```python
from build123d import *

# Parameters (mm, degrees)
F0_W     = 444.5
F0_H     = 654.05
F1_DEPTH = 1092.2
F2_W     = 381
F2_H     = 304.8
F3_DEPTH = 654.05
F5_DEPTH = 304.801
F7_DEPTH = 482.6


# Not quite as in the source:
# - a pattern or mirror of a feature is missing from the dataset's text; its kind, count and spacing are read off the source's solid


with BuildPart() as f1:
    # F0 (on Top) → F1 (new body)
    with BuildSketch(Plane.XY):
        Rectangle(F0_W, F0_H)
    extrude(amount=F1_DEPTH)

    # F2 (on face) → F3 (join, through all)
    with BuildSketch(Plane.XZ.offset(327.025)):
        with Locations((412.75, 152.4)):
            Rectangle(F2_W, F2_H)
        with Locations((-412.75, 152.4)):
            Rectangle(F2_W, F2_H)
    extrude(amount=-F3_DEPTH)

    # F4 (on face) → F5 (cut, through all)
    with BuildSketch(Plane.XY.offset(304.8)):
        Polygon((-314.325, -234.95), (-314.325, 168.9629166667), (-511.175, -168.9629166667), (-511.175, -234.95), align=None)
        Polygon((-511.175, -168.9629166667), (-314.325, 168.9629166667), (-314.325, 234.95), (-511.175, 234.95), align=None)
    f5 = extrude(amount=-F5_DEPTH, mode=Mode.SUBTRACT)

    # F5_copies: F5 across plane
    add(f5.mirror(Plane(origin=(0, 0, 0), x_dir=(0, 0, 1), z_dir=(1, 0, 0))), mode=Mode.SUBTRACT)

    # F6 (on face) → F7 (cut)
    with BuildSketch(Plane.XZ.offset(327.025)):
        with BuildLine():
            ThreePointArc((82.55, 920.75), (58.3716647869, 979.121664787), (0, 1003.3))
            Line((0, 1003.3), (0, 920.75))
            Line((0, 920.75), (82.55, 920.75))
        make_face()
        with BuildLine():
            Line((0, 920.75), (0, 1003.3))
            ThreePointArc((0, 1003.3), (-58.371664787, 979.1216647869), (-82.55, 920.75))
            Line((-82.55, 920.75), (0, 920.75))
        make_face()
        with BuildLine():
            Line((82.55, 920.75), (0, 920.75))
            Line((0, 920.75), (0, 838.2))
            ThreePointArc((0, 838.2), (58.3716647869, 862.378335213), (82.55, 920.75))
        make_face()
        with BuildLine():
            Line((0, 838.2), (0, 920.75))
            Line((0, 920.75), (-82.55, 920.75))
            ThreePointArc((-82.55, 920.75), (-58.371664787, 862.3783352131), (0, 838.2))
        make_face()
        with BuildLine():
            Line((82.55, 787.4), (82.55, 920.75))
            ThreePointArc((82.55, 920.75), (58.3716647869, 862.378335213), (0, 838.2))
            Line((0, 838.2), (0, 787.4))
            Line((0, 787.4), (82.55, 787.4))
        make_face()
        with BuildLine():
            ThreePointArc((0, 838.2), (-58.371664787, 862.3783352131), (-82.55, 920.75))
            Line((-82.55, 920.75), (-82.55, 787.4))
            Line((-82.55, 787.4), (0, 787.4))
            Line((0, 787.4), (0, 838.2))
        make_face()
    extrude(amount=-F7_DEPTH, mode=Mode.SUBTRACT)


solid = f1.part
```
Geometry: final body of the model. Coordinates: model frame, mm. A direction names the side the tool comes from. Round coordinates to 2 decimals unless told otherwise and drop trailing zeros. Order: outer loops, then holes, each group sorted by start corner. A loop starts at its lowest first (then second) coordinate and runs counter-clockwise, first axis right, second up. Notation, with made-up numbers: (79, 11) -> (138, 11) arc R15 ccw to (138, 26) -> close; hole circle Ø3 at (52.25, 68.25). An arc over 180 degrees is marked (long way). Use CSV: the item, a comma, the result in double quotes. Start each with the question number.
1) First-contact query: pin 1 Ø12 at (y, z) = (-214.5, 953.5) entering from -X; pin 2 Ø5 at (x, y) = (243.5, -223) entering from -Z; pin 3 Ø8 at (x, y) = (-320.5, -173.5) entering from -Z. Flat tips, straight axial feed; report the tip coordinate or a pass-through.
2) Set-up query: faces 5 (the face through (-8, -5, 0)), 6 (the face through (-8, 327.025, 432)), 7 (the face through (-288, -5, 304.8)), 8 (the face through (82.55, -89, 853)), 9 (the face through (511.175, 3, 155)). Return all of +Z, -Z, +X, -X, +Y, -Y with unobstructed straight access to the full face (end or side cutting, diameter ignored); none if empty.
3) Draft query along Z for faces 1 (the face through (-603.25, -5, 150)), 2 (the face through (537, -5, 304.8)), 3 (the face through (1.82, -89.1, 1003.28)), 4 (the face through (-1, 155.575, 897)). Return one class per face: +Z half, -Z half, draft (parallel to the pull), parting line (faces both ways), or undercut.
4) Section C-C (x = 0). Return the cut outline in (y, z) (3 decimals), and give its area (3 significant figures).
5) Section D-D (z = 870.5). Return the cut outline in (x, y) (3 decimals).
6) Section B-B (x = 363). Return the cut outline in (y, z) (3 decimals), and give its area (3 significant figures).
7) Material intervals for line 1 along X through (y, z) = (102, 138.5) (3 decimals); line 2 along X through (y, z) = (-251.5, 868.5); line 3 along X through (y, z) = (-219, 357.5), sorted ascending. Write a range as from..to.
8) Section A-A (y = 67). Return the cut outline in (x, z) (3 decimals), and give its area (3 significant figures).
Returned:
1,pin 1,"stops at x = -222.25"
1,pin 2,"stops at z = 0"
1,pin 3,"passes through"
2,face 5,"-Z, +X, -X, +Y, -Y"
2,face 6,"+Z, -Z, +X, -X, +Y"
2,face 7,"+Z, -X, +Y, -Y"
2,face 8,"-Y"
2,face 9,"+Z, -Z"
3,face 1,"draft"
3,face 2,"+Z half"
3,face 3,"undercut"
3,face 4,"undercut"
4,outline,"(-327.025, 0) -> (327.025, 0) -> (327.025, 1092.2) -> (-327.025, 1092.2) -> (-327.025, 1003.3) -> (155.575, 1003.3) -> (155.575, 787.4) -> (-327.025, 787.4) -> close"
4,area,"610,000 mm²"
5,outline,"(-222.25, -327.025) -> (-82.55, -327.025) -> (-82.55, 155.575) -> (82.55, 155.575) -> (82.55, -327.025) -> (222.25, -327.025) -> (222.25, 327.025) -> (-222.25, 327.025) -> close"
6,outline,"(-327.025, 0) -> (-234.95, 0) -> (-234.95, 304.8) -> (-327.025, 304.8) -> close; (234.95, 0) -> (327.025, 0) -> (327.025, 304.8) -> (234.95, 304.8) -> close"
6,area,"56,100 mm²"
7,line 1,"x = -603.25..-511.175, -314.325..314.325, 511.175..603.25"
7,line 2,"x = -222.25..-82.55, 82.55..222.25"
7,line 3,"x = -222.25..222.25"
8,outline,"(-603.25, 0) -> (-511.175, 0) -> (-511.175, 304.8) -> (-603.25, 304.8) -> close; (-314.325, 0) -> (314.325, 0) -> (314.325, 304.8) -> (222.25, 304.8) -> (222.25, 1092.2) -> (-222.25, 1092.2) -> (-222.25, 304.8) -> (-314.325, 304.8) -> close; (511.175, 0) -> (603.25, 0) -> (603.25, 304.8) -> (511.175, 304.8) -> close; hole (-82.55, 787.4) -> (82.55, 787.4) -> (82.55, 920.75) arc R82.55 ccw to (-82.55, 920.75) -> close"
8,area,"565,000 mm²"
